Answer from the drawing. Dimensions are ordinates in mm from the lowest x, y and z of the part. Coordinates: 2 decimals unless noted, no trailing zeros. Order: outer loops, then holes, each group sorted by start corner. A loop starts at its lowest first (then second) coordinate and runs counter-clockwise, first axis right, second up. Notation, with made-up numbers: M 30.25,65.25 L 78.25,65.25 A30 ccw 78.25,103.25 Z; hole C -17.5,9.5 d4. An arc over 180 degrees is marked long. Write each question's results on one line, items separated by ' | '.
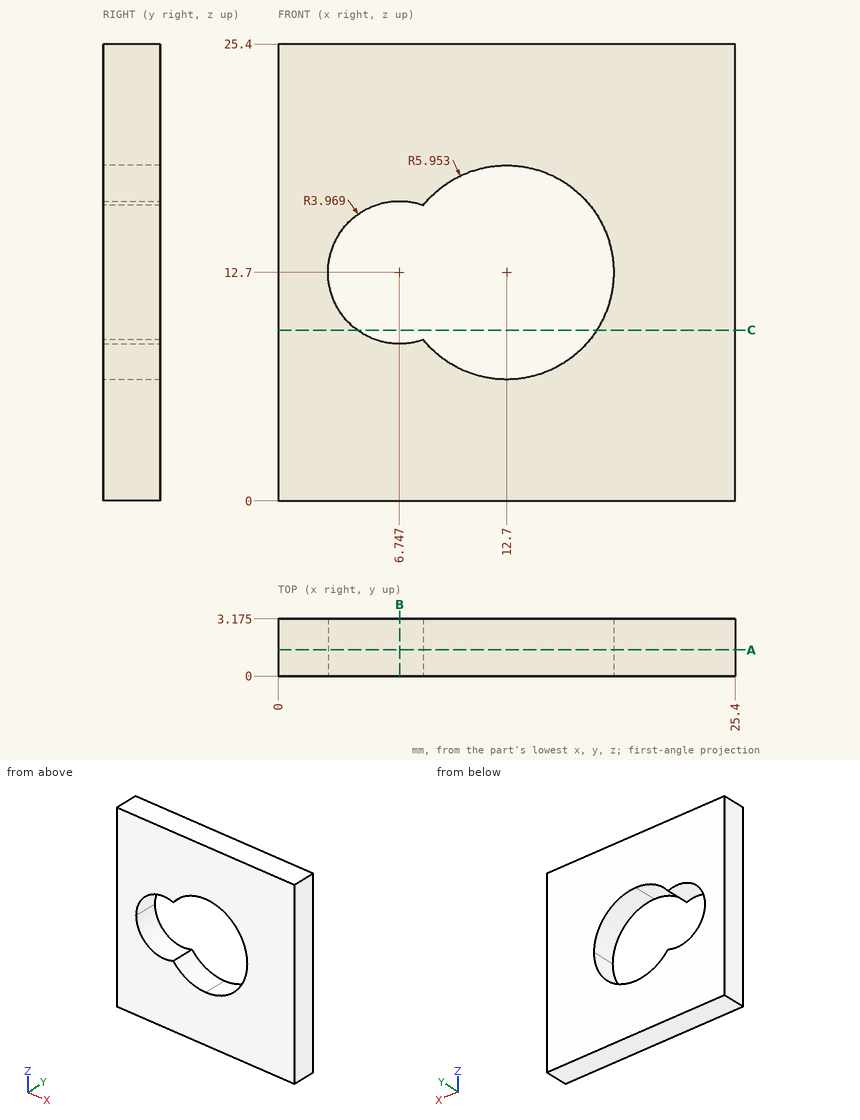
(1) The part is cut by section B-B, the plane x = 6.75. Write down the section's boundary in (y, z) (1 decimal).
Conclusion:
outline: M 0,0 L 3.2,0 L 3.2,8.7 L 0,8.7 Z; M 0,16.7 L 3.2,16.7 L 3.2,25.4 L 0,25.4 Z
(2) The part is cut by section A-A, the plane y = 1.45. Write down the section's boundary in (x, z).
Conclusion:
outline: M 0,0 L 25.4,0 L 25.4,25.4 L 0,25.4 Z; hole M 8.07,8.96 A5.95 ccw long 8.07,16.44 A3.97 ccw long Z
(3) The part is cut by section C-C, the plane z = 9.5. Write down the section's boundary in (x, y) (1 decimal).
Conclusion:
outline: M 0,0 L 4.4,0 L 4.4,3.2 L 0,3.2 Z; M 17.7,0 L 25.4,0 L 25.4,3.2 L 17.7,3.2 Z
(4) Straight lines are drawn through the part: line 1 (Z direction, x = 12.75, y = 0.8); line 2 (X direction, y = 0.65, z = 10.25) (1 decimal). For each, find the intervals that lie inside material, in ascending order.
Conclusion:
line 1: 0 to 6.75, 18.65 to 25.4 | line 2: 0 to 3.6, 18.1 to 25.4
